Geometry check sheet. Reference: the model listing, model coordinates, mm. Face numbers are marked on the shaded views. A direction names the side the tool comes from. Round coordinates to 2 decimals unless told otherwise and drop trailing zeros. Order: outer loops, then holes, each group sorted by start corner. A loop starts at its lowest first (then second) coordinate and runs counter-clockwise, first axis right, second up.
(1) Cross-section at B-B on y = 3.5. Enter the section's corners in (x, z).
(2) Set-up check for the marked faces 4, 5 and 6: record each of +Z, -Z, +X, -X, +Y, -Y from which the full face is reachable in a straight line by a thin tool's end or side.
(3) Draft check along X on the marked faces 1, 2 and 3. Enter one of: pulls with the +X half, pulls with the -X half, needs draft (parallel to the pull), parting line crosses it, or undercut.
(4) Thickness scan on L1, parallel to Z at x = 25, y = 4.5; L2, parallel to Y at x = 16.5, z = -8.5; L3, parallel to Z at x = 26.5, y = 10.5. Record the ranges inside material, lowest first.
(5) Cross-section at C-C on z = -14. Enter the section's corners in (x, y).
(6) Cross-section at D-D on x = 20. Enter the section's corners in (y, z), and give its area (3 significant figures).
(7) Cross-section at A-A on y = 11. Enter the section's corners in (x, z).
(8) Gauge pin test, flat ends, axial feed: P1, Ø6, axis at x = 8, y = 6.5, coming from the -Z side; P2, Ø4.5, axis at x = 17, z = -25.5, coming from the +Y side; P3, Ø5, axis at x = 3.69, z = -3.69, coming from the +Y side; P4, Ø2, axis at x = 18.5, y = 27, coming from the -Z side. Record the tip position at first contact, or that the pin passes through.
Autodesk Inventor part; units mm, degrees
ref_plane "YZ Plane" through (0, 0, 0) normal (1, 0, 0) x (0, 1, 0)
ref_plane "XZ Plane" through (0, 0, 0) normal (0, 1, 0) x (-1, 0, 0)
ref_plane "XY Plane" through (0, 0, 0) normal (0, 0, 1) x (1, 0, 0)
sketch "スケッチ1" plane through (0, 0, 0) normal (0, 1, 0) x (-1, 0, 0)
  line L0 (0, 0) -> (-30, 0)
  line L1 (-30, 0) -> (-30, -30)
  line L2 (-30, -30) -> (0, -30)
  line L3 (0, -30) -> (0, 0)
  dimension "d0" = 30
  dimension "d1" = 30
extrude "押し出し1" add sketch "スケッチ1" along normal blind 5
sketch "スケッチ2" plane through (0, 5, 0) normal (0, 1, 0) x (1, 0, 0)
  line L0 (30, 0) -> (30, 30)
  line L1 (30, 30) -> (0, 30)
  line L2 (0, 30) -> (30, 0) construction
  line L3 (30, 30) -> (0, 0) construction
  circle A0 centre (15, 15) radius 16 construction
  point P0 (26.3137, 26.3137)
  point P1 (26.3137, 3.6863)
  point P2 (3.6863, 3.6863)
  point P3 (3.6863, 26.3137)
  point P4 (15, 15)
  dimension "d12" = 32
  dimension "d76" = 0
hole "穴2" at (26.3137, 5, -26.3137) at (26.3137, 5, -3.6863) at (3.6863, 5, -3.6863) at (3.6863, 5, -26.3137) direction (0, -1, 0) diameter 3.2 end through all
sketch "スケッチ3" plane through (0, 5, 0) normal (0, 1, 0) x (1, 0, 0)
  circle A0 centre (26.3137, 3.6863) radius 1.6
  circle A1 centre (3.6863, 3.6863) radius 1.6
  circle A2 centre (3.6863, 26.3137) radius 1.6
  circle A3 centre (26.3137, 26.3137) radius 1.6
  point P0 (0, 0)
hole "穴3" at (26.3137, 5, -3.6863) at (3.6863, 5, -3.6863) at (3.6863, 5, -26.3137) at (26.3137, 5, -26.3137) direction (0, -1, 0) diameter 5.8 depth 3 tip angle 118
sketch "スケッチ4" plane through (0, 5, 0) normal (0, 1, 0) x (1, 0, 0)
  line L0 (0, 30) -> (0, 0)
  line L1 (30, 0) -> (30, 30)
  line L2 (0, 7) -> (30, 7)
  line L3 (30, 7) -> (30, 23)
  line L4 (30, 23) -> (0, 23)
  line L5 (0, 23) -> (0, 7)
  line L6 (0, 0) -> (30, 0)
  point P0 (0, 23)
  dimension "d27" = 16
  dimension "d28" = 7
extrude "押し出し2" add sketch "スケッチ4" along normal blind 35 contours L4 L1 L2 L0
fillet "フィレット6" radius 2 4 edges at (30, 2.5, 0) (0, 2.5, 0) (0, 2.5, -30) (30, 2.5, -30)
sketch "スケッチ8" plane through (0, 5, -7) normal (0, 0, 1) x (1, 0, 0)
  line L0 (0, 35) -> (30, 35)
  line L1 (2, 0) -> (28, 0)
  point P0 (0, -5)
  point P1 (15, 6)
  point P2 (15, 35)
  point P3 (3.089, 0)
  point P4 (23.911, 0)
  dimension "d61" = 6
hole "穴6" at (15, 11, -7) direction (0, 0, -1) diameter 6.5 end through all
fillet "フィレット7" [suppressed]
fillet "フィレット8" radius 0.1 2 edges at (15, 5, -23) (15, 5, -7)
fillet "フィレット9" radius 1 22 edges at (15, 40, -23) (15, 40, -7) (30, 5.0293, -23.0293) (30, 5, -25.55) (29.4142, 5, -29.4142) (15, 5, -30) (0.5858, 5, -29.4142) (0, 5, -25.55) (0, 5.0293, -23.0293) (0, 22.55, -23) (30, 22.55, -23) (0, 5.0293, -6.9707) (0, 5, -4.45) (0.5858, 5, -0.5858) (15, 5, 0) (29.4142, 5, -0.5858) (30, 5, -4.45) (30, 5.0293, -6.9707) (30, 22.55, -7) (0, 22.55, -7) (30, 40, -15) (0, 40, -15)
fillet "フィレット10" [suppressed]
sketch "スケッチ10" plane through (29, 5.1, -23) normal (0, 0, -1) x (-1, 0, 0)
  line L0 (0, 34.9) -> (28, 34.9) construction
  circle A0 centre (14, 5.9) radius 3.25 construction
  line L1 (14, 34.9) -> (14, 5.9) construction
  arc A1 (9, 33.9) -> (0, 24.9) centre (9, 24.9) ccw construction
  line L2 (14, 5.9) -> (10.7733, 32.1791) construction
  circle A2 centre (14, 5.9) radius 20 construction
  point P0 (29, -5.1)
  point P1 (9, 34.9)
  point P2 (19, 34.9)
  point P3 (11.5626, 25.7509)
  point P4 (-1, 34.9)
  point P5 (29, 34.9)
  dimension "d85" = 40
  dimension "d84" = 7
hole "穴7" at (17.4374, 30.8509, -23) direction (0, 0, 1) diameter 6.5 end through all
properties part number "NewPart2"
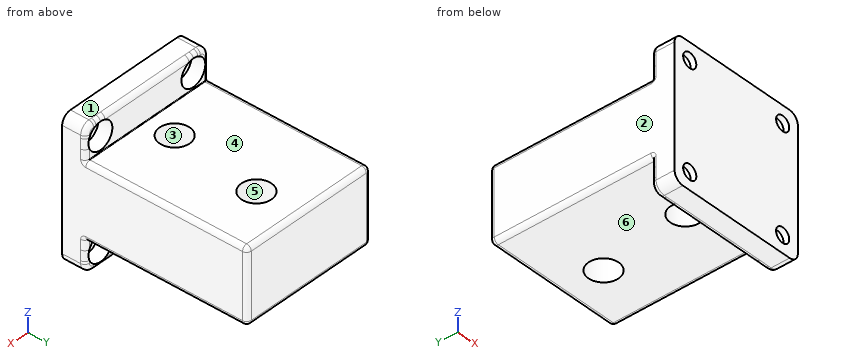
Found:
1. outline: (0, -28) arc R2 ccw to (2, -30) - (28, -30) arc R2 ccw to (30, -28) - (30, -2) arc R2 ccw to (28, 0) - (2, 0) arc R2 ccw to (0, -2) - close; hole circle Ø5.8 at (3.69, -26.31); hole circle Ø5.8 at (3.69, -3.69); hole circle Ø5.8 at (26.31, -26.31); hole circle Ø5.8 at (26.31, -3.69)
2. face 4: +Z, +X, -X, +Y
2. face 5: +Z, -Z
2. face 6: -Z, +X, -X, +Y
3. face 1: needs draft
3. face 2: pulls with the -X half
3. face 3: undercut
4. L1: z = -29.87 to -28.9, -23.73 to -6.27, -1.1 to -0.13
4. L2: y = 0 to 8.12, 13.88 to 27.74, 33.96 to 40
4. L3: z = -23 to -7
5. outline: (0, 0) - (30, 0) - (30, 39) arc R1 ccw to (29, 40) - (1, 40) arc R1 ccw to (0, 39) - close; hole circle Ø6.5 at (15, 11); hole circle Ø6.5 at (17.44, 30.85)
6. outline: (0, -30) - (4, -30) arc R1 ccw to (5, -29) - (5, -23.1) arc R0.1 cw to (5.1, -23) - (28.85, -23) - (28.85, -7) - (5.1, -7) arc R0.1 cw to (5, -6.9) - (5, -1) arc R1 ccw to (4, 0) - (0, 0) - close; (32.85, -23) - (39, -23) arc R1 ccw to (40, -22) - (40, -8) arc R1 ccw to (39, -7) - (32.85, -7) - close
6. area: 645 mm2
7. outline: (0, -22) arc R1 ccw to (1, -23) - (11.75, -23) - (11.75, -7) - (1, -7) arc R1 ccw to (0, -8) - close; (18.25, -23) - (29, -23) arc R1 ccw to (30, -22) - (30, -8) arc R1 ccw to (29, -7) - (18.25, -7) - close
8. P1: stops at z = -30
8. P2: stops at y = 5
8. P3: stops at y = 1.76
8. P4: stops at z = -23
